Source: CAD feature listing. Evaluate the final solid. Frame: model axes, mm. Face numbers are marked on the shaded views. A direction names the side the tool comes from. Give positions to 0.01 mm unless a question says otherwise; leave off trailing zeros. Order: outer loops, then holes, each group sorted by start corner. A loop starts at its lowest first (then second) coordinate and runs counter-clockwise, first axis right, second up.
from build123d import *

# Parameters (mm, degrees)
BOSS_EXTRU_1_DEPTH = 15
ESQUISSE5_W        = 200
ESQUISSE5_H        = 10
BOSS_EXTRU_4_DEPTH = 6
BOSS_EXTRU_5_DEPTH = 12
BOSS_EXTRU_6_DEPTH = 12


with BuildPart() as part:
    # Esquisse1 → Boss.-Extru.1 (new body)
    with BuildSketch(Plane.XY):
        Polygon((-29.902548443, 15.22370444), (-6.802548443, 15.22370444), (25.697451557, -41.067946806), (25.697451557, -58.033349019), (19.697451557, -58.033349019), (19.697451557, -48.033349019), (-9.895822056, 3.22370444), (-29.902548443, 3.22370444), align=None)
    extrude(amount=BOSS_EXTRU_1_DEPTH)

    # Esquisse5 → Boss.-Extru.4 (add)
    with BuildSketch(Plane(origin=(25.697451557, 0, 0), x_dir=(0, 0, -1), z_dir=(1, 0, 0))):
        with Locations((-7.5, -53.033349019)):
            Rectangle(ESQUISSE5_W, ESQUISSE5_H)
    extrude(amount=-BOSS_EXTRU_4_DEPTH)

    # Esquisse6 → Boss.-Extru.5 (add)
    with BuildSketch(Plane(origin=(0, 15.22370444, 0), x_dir=(1, 0, 0), z_dir=(0, 1, 0))):
        Polygon((-29.902548443, -15), (-9.895822056, -15), (-29.902548443, -21.702554703), align=None)
    extrude(amount=-BOSS_EXTRU_5_DEPTH)

    # Esquisse7 → Boss.-Extru.6 (add)
    with BuildSketch(Plane(origin=(0, 15.22370444, 0), x_dir=(1, 0, 0), z_dir=(0, 1, 0))):
        Polygon((-29.902548443, 0), (-9.895822056, 0), (-29.902548443, 6.692394801), align=None)
    extrude(amount=-BOSS_EXTRU_6_DEPTH)


solid = part.part
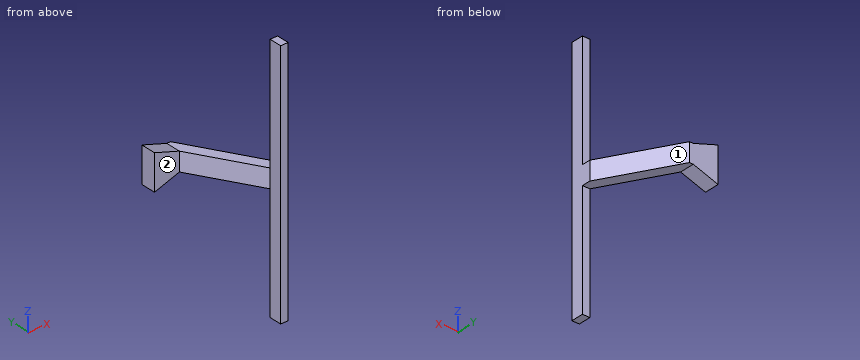
1) Section query A-A on y = -52. Output: boundary loops of the cut face in (x, z).
Checks:
outline: (19.7, -92.5) - (25.7, -92.5) - (25.7, 107.5) - (19.7, 107.5) - close
2) Reachability of the marked faces 1 and 2 from +Z, -Z, +X, -X, +Y, -Y: full face, straight path, thin tool, end or side. Return the list, or none.
Checks:
face 1: +Z, -Z, +X, +Y
face 2: +Z, -Z, -X, -Y
3) Section query C-C on y = 10.5. Output: boundary loops of the cut face in (x, z).
Checks:
outline: (-29.9, -6.69) - (-9.9, 0) - (-4.08, 0) - (-4.08, 15) - (-9.9, 15) - (-29.9, 21.7) - close
4) Section query B-B on x = 9. Output: boundary loops of the cut face in (y, z).
Checks:
outline: (-29.5, 0) - (-12.15, 0) - (-12.15, 15) - (-29.5, 15) - close
5) Ray query, L1, parallel to Z at x = 3, y = -13.5; L2, parallel to Y at x = 11.5, z = 5.5; L3, parallel to X at y = -32.5, z = 10. Return the intervals inside material, ascending.
Checks:
L1: z = 0 to 15
L2: y = -33.83 to -16.48
L3: x = 10.73 to 20.75
6) First-contact query: pin 1 Ø5 at (y, z) = (-22, 2) entering from -X; pin 2 Ø3 at (y, z) = (-50.5, 13) entering from -X; pin 3 Ø1.8 at (x, z) = (24, -33) entering from +Y. Flat tips, straight axial feed; report the tip coordinate or a pass-through.
Checks:
pin 1: stops at x = 3.22
pin 2: stops at x = 19.7
pin 3: stops at y = -48.03
